Here's the drawing with two shaded views (mm, measured from the low corner). I have some questions. A direction names the side the tool comes from. Round coordinates to 2 decimals unless told otherwise and drop trailing zeros. Loops run counter-clockwise (first coordinate to the right, second up) from the corner with the lowest first, then second, coordinate; pieces in that order, holes last. Notation, with made-up numbers: (55.5, 70) -> (80.5, 70) arc R17 cw to (80.5, 87) -> close; hole circle Ø10 at (73, 44.25). An arc over 180 degrees is marked (long way). Use a Markdown table: item, result.
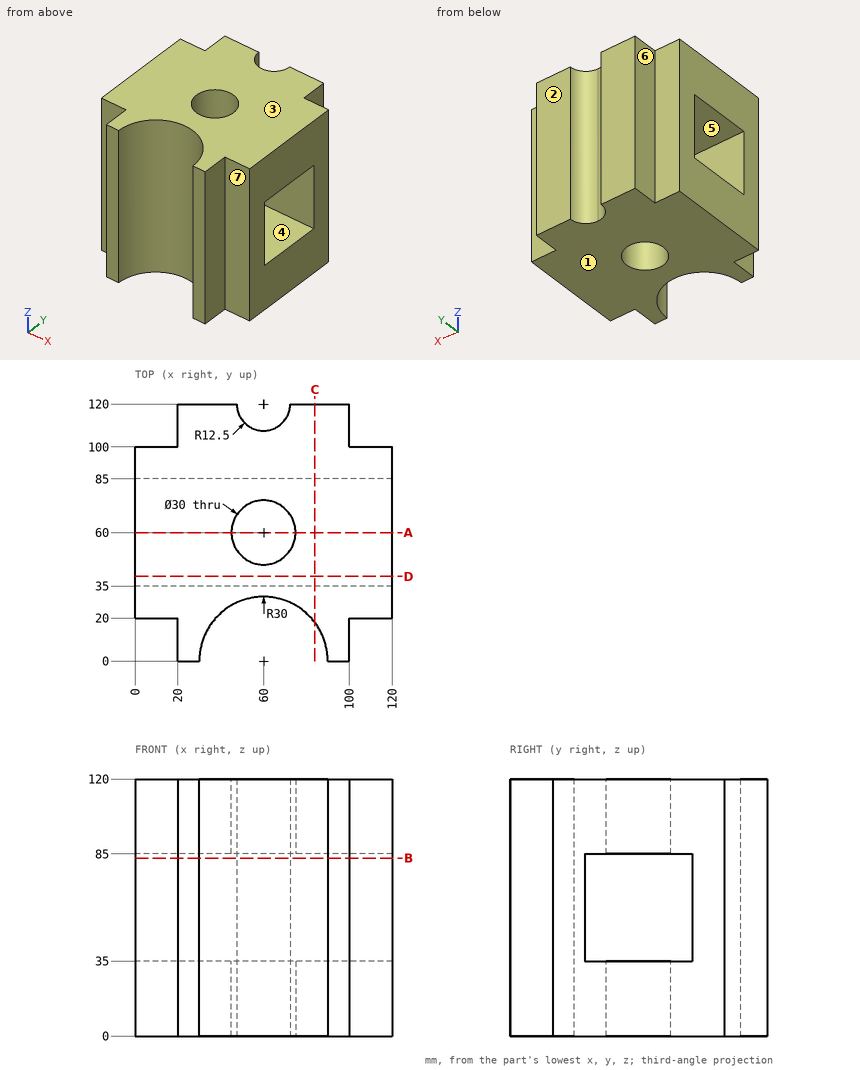
1. I need wall thicknesses on line 1 (Z direction, x = 18.5, y = 48); line 2 (Y direction, x = 113.5, z = 72); line 3 (Y direction, x = 60, z = 15.5). Which ranges of each line are inside material? Lowest first, please.
Answer sheet:
| item | result |
|---|---|
| line 1 | z = 0 to 35, 85 to 120 |
| line 2 | y = 20 to 35, 85 to 100 |
| line 3 | y = 30 to 45, 75 to 107.5 |
2. I want a section at B-B (z = 83). Please give me the cut outline in (x, y).
Answer sheet:
| item | result |
|---|---|
| outline | (0, 20) -> (20, 20) -> (20, 0) -> (30, 0) arc R30 cw to (90, 0) -> (100, 0) -> (100, 20) -> (120, 20) -> (120, 35) -> (0, 35) -> close; (0, 85) -> (120, 85) -> (120, 100) -> (100, 100) -> (100, 120) -> (72.5, 120) arc R12.5 cw to (47.5, 120) -> (20, 120) -> (20, 100) -> (0, 100) -> close |
3. If we mould it in two halves opening along Z, with no side actions, what happens to the marked faces 1, 2, 3 and 4? For each: +Z half, -Z half, draft (parallel to the pull), parting line (faces both ways), or undercut.
Answer sheet:
| item | result |
|---|---|
| face 1 | -Z half |
| face 2 | draft |
| face 3 | +Z half |
| face 4 | undercut |
4. Will these pins go through, and if not, where does the flat tip stop? pin 1 Ø16 at (x, z) = (108.5, 47.5) entering from +Y; pin 2 Ø10 at (x, z) = (109, 80) entering from -Y; pin 3 Ø10 at (y, z) = (112, 83) entering from +X.
Answer sheet:
| item | result |
|---|---|
| pin 1 | stops at y = 100 |
| pin 2 | stops at y = 20 |
| pin 3 | stops at x = 100 |
5. I want a section at C-C (x = 84). Please give me the cut outline in (y, z).
Answer sheet:
| item | result |
|---|---|
| outline | (18, 0) -> (120, 0) -> (120, 120) -> (18, 120) -> close; hole (35, 35) -> (85, 35) -> (85, 85) -> (35, 85) -> close |
6. I want a section at D-D (y = 39.5). Please give me the cut outline in (x, z).
Answer sheet:
| item | result |
|---|---|
| outline | (0, 0) -> (120, 0) -> (120, 35) -> (0, 35) -> close; (0, 85) -> (120, 85) -> (120, 120) -> (0, 120) -> close |
7. I want a section at A-A (y = 60). Please give me the cut outline in (x, z), plus the area to 3 significant figures.
Answer sheet:
| item | result |
|---|---|
| outline | (0, 0) -> (45, 0) -> (45, 35) -> (0, 35) -> close; (0, 85) -> (45, 85) -> (45, 120) -> (0, 120) -> close; (75, 0) -> (120, 0) -> (120, 35) -> (75, 35) -> close; (75, 85) -> (120, 85) -> (120, 120) -> (75, 120) -> close |
| area | 6,300 mm² |
8. Which directions (+Z, -Z, +X, -X, +Y, -Y) give clear straight access to the entire face, cutting with the end or side of a thin tool? Please do the marked faces 5, 6 and 7.
Answer sheet:
| item | result |
|---|---|
| face 5 | +X, -X |
| face 6 | +Z, -Z, -X, +Y |
| face 7 | +Z, -Z, +X, -Y |
